Source: CAD feature listing. Evaluate the final solid. Frame: model axes, mm. A direction names the side the tool comes from. Coordinates: 2 decimals unless noted, no trailing zeros. Order: outer loops, then holes, each group sorted by start corner. A loop starts at its lowest first (then second) coordinate and runs counter-clockwise, first axis right, second up. Notation, with made-up numbers: (-5, 72) - (26, 72) arc R21 ccw to (26, 94) - close; hole circle Ø3 at (71, 84.25). An arc over 180 degrees is marked (long way). One line per question, with ' | ' between items.
from build123d import *

# Parameters (mm, degrees)
F0_W     = 33.416076
F0_H     = 33.374747
F0_R     = 15.588949
F1_DEPTH = 25.4
F3_DEPTH = 25.4


with BuildPart() as f1:
    # F0 (on Top) → F1 (new body)
    with BuildSketch(Plane.XY):
        with Locations((-33.761238, 29.984143)):
            Rectangle(F0_W, F0_H)
        with Locations((-33.995453, 29.879961)):
            Circle(F0_R, mode=Mode.SUBTRACT)
    extrude(amount=F1_DEPTH)

    # F2 (on Top) → F3 (join)
    with BuildSketch(Plane.XY):
        Polygon((-20.725947, 20.616256), (-33.770509, 45.134839), (-46.487864, 20.616256), align=None)
    extrude(amount=F3_DEPTH)


solid = f1.part
(1) Cut plane D-D (y = 39). Return the cut outline in (x, z).
Taken from the geometry:
outline: (-50.47, 0) - (-46.64, 0) - (-46.64, 25.4) - (-50.47, 25.4) - close; (-36.95, 0) - (-30.51, 0) - (-30.51, 25.4) - (-36.95, 25.4) - close; (-21.35, 0) - (-17.05, 0) - (-17.05, 25.4) - (-21.35, 25.4) - close
(2) Material intervals for L1, parallel to X at y = 22.5, z = 17.25; L2, parallel to X at y = 37, z = 8.75; L3, parallel to Y at x = -38, z = 3, sorted ascending. Write a range as from..to.
Taken from the geometry:
L1: x = -50.47..-47.73, -45.51..-21.73, -20.26..-17.05 | L2: x = -50.47..-47.86, -37.99..-29.44, -20.13..-17.05 | L3: y = 13.3..14.81, 20.62..36.98, 44.95..46.67
(3) Cut plane B-B (x = -41). Return the cut outline in (y, z), and give its area (3 significant figures).
Taken from the geometry:
outline: (13.3, 0) - (15.95, 0) - (15.95, 25.4) - (13.3, 25.4) - close; (20.62, 0) - (31.2, 0) - (31.2, 25.4) - (20.62, 25.4) - close; (43.81, 0) - (46.67, 0) - (46.67, 25.4) - (43.81, 25.4) - close | area: 409 mm²
(4) Cut plane C-C (y = 17.5). Return the cut outline in (x, z).
Taken from the geometry:
outline: (-50.47, 0) - (-43.47, 0) - (-43.47, 25.4) - (-50.47, 25.4) - close; (-24.52, 0) - (-17.05, 0) - (-17.05, 25.4) - (-24.52, 25.4) - close
(5) Set-up query: faces 1 (the flat face through (-34, 20.616, 13)), 2 (the flat face through (-34, 46.672, 13)). Return all of +Z, -Z, +X, -X, +Y, -Y with unobstructed straight access to the full face (end or side cutting, diameter ignored); none if empty.
Taken from the geometry:
face 1: +Z, -Z | face 2: +Z, -Z, +X, -X, +Y
(6) Pull-direction query (X, two-part tool) for faces 3 (the flat face through (-27.317, 33.004, 12.522)), 4 (the flat face through (-34, 30, 25.4)), 5 (the flat face through (-17.053, 30, 13)); classes: pulls with the +X half, pulls with the -X half, needs draft (parallel to the pull), parting line crosses it, or undercut.
Taken from the geometry:
face 3: undercut | face 4: needs draft | face 5: pulls with the +X half
(7) Cut plane A-A (z = 7). Return the cut outline in (x, y).
Taken from the geometry:
outline: (-50.47, 13.3) - (-17.05, 13.3) - (-17.05, 46.67) - (-50.47, 46.67) - close; hole (-46.49, 20.62) - (-33.77, 45.13) - (-21.04, 21.21) arc R15.59 ccw (long way) to (-21.46, 20.62) - close
